```python
from build123d import *
from build123d.topology import SkipClean

# Parameters (mm, degrees)
SKETCH1_R           = 10.5
SKETCH1_R_2         = 8.6
BOSS_EXTRUDE1_DEPTH = 2
SKETCH2_W           = 0.8
SKETCH2_H           = 1.25
BOSS_EXTRUDE2_DEPTH = 1.25
BOSS_EXTRUDE3_START = 17.2
SKETCH2_2_W         = 0.8
SKETCH2_2_H         = 1.25
BOSS_EXTRUDE3_DEPTH = 1.25
BOSS_EXTRUDE4_START = 0.5
SKETCH3_R           = 10.5
BOSS_EXTRUDE4_DEPTH = 0.5
SKETCH5_R           = 3.25
BOSS_EXTRUDE5_DEPTH = 6
FILLET2_R           = 0.75
CUT_EXTRUDE1_DEPTH  = 5.5
FILLET1_R           = 0.25
SKETCH7_R           = 2.625
CUT_EXTRUDE2_DEPTH  = 2.5
CUT_EXTRUDE3_DEPTH  = 0.25
SKETCH11_R          = 2.5
BOSS_EXTRUDE6_DEPTH = 5
CUT_EXTRUDE4_START  = 5
CUT_EXTRUDE4_DEPTH  = 4.5
CHAMFER2_SIZE       = 0.25
FILLET3_R           = 5


with BuildPart() as part:
    # Sketch1 → Boss-Extrude1 (new body)
    with BuildSketch(Plane(origin=(0, 0, 0), x_dir=(1, 0, 0), z_dir=(0, 1, 0))):
        with Locations(Location((0, 0, 0), (0, 0, 270))):
            Circle(SKETCH1_R)
        with Locations(Location((0, 0, 0), (0, 0, 270))):
            Circle(SKETCH1_R_2, mode=Mode.SUBTRACT)
    extrude(amount=-BOSS_EXTRUDE1_DEPTH)

    # Sketch2 → Boss-Extrude2 (add)
    with BuildSketch(Plane(origin=(0, 0, 8.6), x_dir=(-1, 0, 0), z_dir=(0, 0, -1))):
        with Locations((0, -0.625)):
            Rectangle(SKETCH2_W, SKETCH2_H)
    extrude(amount=BOSS_EXTRUDE2_DEPTH)

    # Sketch2<2> → Boss-Extrude3 (add)
    with BuildSketch(Plane(origin=(0, 0, 8.6), x_dir=(-1, 0, 0), z_dir=(0, 0, -1)).offset(BOSS_EXTRUDE3_START)):
        with Locations((0, -0.625)):
            Rectangle(SKETCH2_2_W, SKETCH2_2_H)
    extrude(amount=-BOSS_EXTRUDE3_DEPTH)

    # Sketch3 → Boss-Extrude4 (add)
    with BuildSketch(Plane(origin=(0, 0, 0), x_dir=(1, 0, 0), z_dir=(0, 1, 0)).offset(BOSS_EXTRUDE4_START)):
        with Locations(Location((0, 0, 0), (0, 0, 270))):
            Circle(SKETCH3_R)
    extrude(amount=-BOSS_EXTRUDE4_DEPTH)

    # Sketch5 → Boss-Extrude5 (add)
    with BuildSketch(Plane.XZ):
        with Locations(Location((0, 0, 0), (0, 0, 90))):
            Circle(SKETCH5_R)
    extrude(amount=BOSS_EXTRUDE5_DEPTH)

    # Fillet2
    fillet2_edges = [part.edges().sort_by_distance(p)[0] for p in [
        (0, 0, -3.25),
    ]]
    fillet(fillet2_edges, radius=FILLET2_R)

    # Sketch4 → Cut-Extrude1 (cut)
    with BuildSketch(Plane(origin=(0, 0.5, 0), x_dir=(1, 0, 0), z_dir=(0, 1, 0))):
        with BuildLine():
            Line((-1.469693846, 2.175), (1.469693846, 2.175))
            ThreePointArc((1.469693846, 2.175), (0, -2.625), (-1.469693846, 2.175))
        make_face()
    extrude(amount=-CUT_EXTRUDE1_DEPTH, mode=Mode.SUBTRACT)

    # Fillet1
    fillet1_edges = [part.edges().sort_by_distance(p)[0] for p in [
        (-0.4, -1.25, 7.970346319),
        (0.4, -1.25, 7.970346319),
        (-0.4, -1.25, -7.970346319),
        (0.4, -1.25, -7.970346319),
    ]]
    fillet(fillet1_edges, radius=FILLET1_R)

    # Sketch7 → Cut-Extrude2 (cut)
    with SkipClean():  # the faces are left unmerged after this step: merging them gives an invalid solid
        with BuildSketch(Plane(origin=(0, 0.5, 0), x_dir=(1, 0, 0), z_dir=(0, 1, 0))):
            with Locations(Location((0, 0, 0), (0, 0, 270))):
                Circle(SKETCH7_R)
        extrude(amount=-CUT_EXTRUDE2_DEPTH, mode=Mode.SUBTRACT)

    # Sketch9 → Cut-Extrude3 (cut)
    with SkipClean():  # the faces are left unmerged after this step: merging them gives an invalid solid
        with BuildSketch(Plane(origin=(0, 0.5, 0), x_dir=(1, 0, 0), z_dir=(0, 1, 0))):
            with BuildLine():
                Line((-0.5, 3.7), (-0.5, 13.7))
                ThreePointArc((-0.5, 13.7), (0, 14.2), (0.5, 13.7))
                Line((0.5, 13.7), (0.5, 3.7))
                ThreePointArc((0.5, 3.7), (0, 3.2), (-0.5, 3.7))
            make_face()
        extrude(amount=-CUT_EXTRUDE3_DEPTH, mode=Mode.SUBTRACT)

    # Sketch11 → Boss-Extrude6 (add)
    with SkipClean():  # the faces are left unmerged after this step: merging them gives an invalid solid
        with BuildSketch(Plane.XZ.offset(6)):
            with Locations(Location((0, 0, 0), (0, 0, 270))):
                Circle(SKETCH11_R)
        extrude(amount=BOSS_EXTRUDE6_DEPTH)

    # Sketch10 → Cut-Extrude4 (cut)
    with SkipClean():  # the faces are left unmerged after this step: merging them gives an invalid solid
        with BuildSketch(Plane.XZ.offset(6).offset(CUT_EXTRUDE4_START)):
            Polygon((1.804219591, 0), (0.902109796, 1.5625), (-0.902109796, 1.5625), (-1.804219591, 0), (-0.902109796, -1.5625), (0.902109796, -1.5625), align=None)
        extrude(amount=-CUT_EXTRUDE4_DEPTH, mode=Mode.SUBTRACT)

    # Chamfer2
    chamfer2_edges = [part.edges().sort_by_distance(p)[0] for p in [
        (-1.353164693, -11, -0.78125),
        (-1.353164693, -11, 0.78125),
        (0, -11, 1.5625),
        (1.353164693, -11, 0.78125),
        (1.353164693, -11, -0.78125),
        (0, -11, -1.5625),
    ]]
    chamfer(chamfer2_edges, length=CHAMFER2_SIZE)

    # Fillet3
    # the kernel refuses this fillet: 5 mm, written as the material it adds along each edge
    with BuildSketch(Plane(origin=(0, -6, 0), x_dir=(0, 0, -1), z_dir=(-1, 0, 0))) as fillet3_piece_1:
        with BuildLine():
            CenterArc((7.5, 2.633913438), FILLET3_R, 180, 31.788330617)
            Line((3.25, 0), (3.165, -0.052678269))
            ThreePointArc((3.165, -0.052678269), (2.875, -0.1), (2.5, -0.1))
            Line((2.5, -0.1), (2.4, 0))
            Line((2.4, 0), (2.4, 2.633913438))
            Line((2.4, 2.633913438), (2.5, 2.633913438))
        make_face()
    revolve(axis=Axis((0, -6, 0), (0, -1, 0)))


solid = part.part
```
Geometry: final body of the model. Coordinates: model frame, mm. A direction names the side the tool comes from. Coordinates: 2 decimals unless noted, no trailing zeros. Order: outer loops, then holes, each group sorted by start corner. A loop starts at its lowest first (then second) coordinate and runs counter-clockwise, first axis right, second up. Notation, with made-up numbers: (69, 35) - (90, 35) arc R27 cw to (90, 63) - close; hole circle Ø7 at (6, -28.5). An arc over 180 degrees is marked (long way). Write each question's results on one line, items separated by ' | '.
(1) Set-up query: faces 1 (the face through (0, -3, -2.175)), 2 (the face through (-2, 0.5, 2)), 3 (the face through (0, -9, -1.562)). Return all of +Z, -Z, +X, -X, +Y, -Y with unobstructed straight access to the full face (end or side cutting, diameter ignored); none if empty.
Values found:
face 1: +Y | face 2: +Z, -Z, +X, -X, +Y | face 3: -Y
(2) Section query C-C, the plane z = 6.75. Return the cut outline in (x, y).
Values found:
outline: (-8.04, -2) - (-5.33, -2) - (-5.33, 0) - (5.33, 0) - (5.33, -2) - (8.04, -2) - (8.04, 0.5) - (-8.04, 0.5) - close
(3) First-contact query: pin 1 Ø6 at (x, y) = (2.5, -9) entering from -Z; pin 2 Ø0.5 at (x, z) = (0.5, -2.5) entering from +Y; pin 3 Ø0.8 at (y, z) = (-0.5, 8) entering from +X (3 decimals); pin 4 Ø2 at (x, y) = (0, -7.5) entering from -Z. Flat tips, straight axial feed; report the tip coordinate or a pass-through.
Values found:
pin 1: stops at z = -2.86 | pin 2: stops at y = 0.5 | pin 3: stops at x = 7.245 | pin 4: stops at z = -2.98
(4) Section query B-B, the plane z = -4.75. Return the cut outline in (x, y).
Values found:
outline: (-9.36, -2) - (-7.17, -2) - (-7.17, 0) - (7.17, 0) - (7.17, -2) - (9.36, -2) - (9.36, 0.5) - (0.5, 0.5) - (0.5, 0.25) - (-0.5, 0.25) - (-0.5, 0.5) - (-9.36, 0.5) - close
(5) Line query: line 1 (X direction, y = -1.5, z = 0) (3 decimals); line 2 (X direction, y = -0.7, z = 0) (3 decimals); line 3 (X direction, y = -3.45, z = 0) (3 decimals). Output: solid intervals per line, ascending. Write a range as [from, to].
Values found:
line 1: x = [-10.5, -8.6], [-3.25, -2.625], [2.625, 3.25], [8.6, 10.5] | line 2: x = [-10.5, -8.6], [-3.252, -2.625], [2.625, 3.252], [8.6, 10.5] | line 3: x = [-3.25, -2.625], [2.625, 3.25]
(6) Section query A-A, the plane y = -7.5. Return the cut outline in (x, z).
Values found:
outline: circle Ø5.26 at (0, 0); hole (-1.8, 0) - (-0.9, -1.56) - (0.9, -1.56) - (1.8, 0) - (0.9, 1.56) - (-0.9, 1.56) - close
